from build123d import *


with BuildPart() as part:
    # Sketch1 → Revolve1 (revolve)
    with BuildSketch(Plane.XY, mode=Mode.PRIVATE) as revolve1_sk:
        Polygon((2.8, 24), (2.8, 22), (6.8, 22), (6.8, 20), (2.8, 20), (2.8, 18), (2.8, 16), (6.8, 16), (6.8, 14), (2.8, 14), (2.8, 12), (2.8, 10), (6.8, 10), (6.8, 8), (2.8, 8), (2.8, 6), (2.8, 4), (6.8, 4), (6.8, 2), (2.8, 2), (2.8, 0), (2.8, -2), (6.8, -2), (6.8, -4), (2.8, -4), (2.8, -6), (2.8, -8), (6.8, -8), (6.8, -10), (2.8, -10), (2.8, -12), (2.8, -14), (6.8, -14), (6.8, -16), (2.8, -16), (2.8, -18), (2.8, -20), (6.8, -20), (6.8, -22), (2.8, -22), (2.8, -24), (4.8, -24), (4.8, -27), (0, -27), (0, 27), (4.8, 27), (4.8, 24), align=None)
    revolve(revolve1_sk.sketch.rotate(Axis((0, 27, 0), (0, -1, 0)), 180), axis=Axis((0, 27, 0), (0, -1, 0)))


solid = part.part
Geometry check sheet. Reference: the model listing, model coordinates, mm. A direction names the side the tool comes from. Give positions to 0.01 mm unless a question says otherwise; leave off trailing zeros. Write each loop counter-clockwise with the first axis right and the second up, starting at its lowest first coordinate (ties: lowest second). Pieces come first, ordered by that corner, then holes. Notation, with made-up numbers: M 69,-22 L 93,-22 A20 cw 93,-3 Z; hole C -33.5,71 d6. An arc over 180 degrees is marked long. One line per question, with ' | ' between items.
1. Cross-section at C-C (y = 1.5). Enter the section's corners in (x, z).
Ans:
outline: C 0,0 d5.6
2. Set-up check for faces 1 (the face through (-2.58, 25.48, -4.05)), 2 (the face through (2.8, 23, -0.1)): record each of +Z, -Z, +X, -X, +Y, -Y from which the full face is reachable in a straight line by a thin tool's end or side.
Ans:
face 1: +Y | face 2: none
3. Mould release check, pull along Y, two halves, no side actions. Record for faces 3 (the face through (-2.58, -25.52, -4.05)), 4 (the face through (2.8, 0, -0.1)): released by +Y, released by -Y, zero draft, split by the parting line, or undercut.
Ans:
face 3: zero draft | face 4: undercut
4. Cross-section at A-A (z = -5.5). Count the separate pieces of the cut face and the enclosed holes in it, plus the area to 3 significant figures.
Ans:
separate pieces: 8 | enclosed holes: 0 | area: 128 mm2
5. Gauge pin test, flat ends, axial feed: pin 1 (3 mm diameter, centred on x = 5, y = 4, fed in from -Z); pin 2 (3 mm diameter, centred on x = -5.5, y = 4, fed in from -Z); pin 3 (4 mm diameter, centred on y = -17.5, z = -4, fed in from +X). Record the tip position at first contact, or that the pin passes through.
Ans:
pin 1: z = -5.83 | pin 2: z = -5.5 | pin 3: x = 6.25
6. Scan lines: line 1 along Z through (x, y) = (0.25, 9); line 2 along X through (y, z) = (21.5, -5.5); line 3 along Z through (x, y) = (0.25, 6). Record each from-to range of solid material in increasing order. Write a range as from..to.
Ans:
line 1: -6.8..6.8 | line 2: -4..4 | line 3: -2.79..2.79
